Part model, mm, in its own coordinate system. A direction names the side the tool comes from. Round coordinates to 2 decimals unless told otherwise and drop trailing zeros. Order: outer loops, then holes, each group sorted by start corner. A loop starts at its lowest first (then second) coordinate and runs counter-clockwise, first axis right, second up. Notation, with made-up numbers: (57, 66) - (94, 66) arc R22 ccw to (94, 102) - close; hole circle Ø10 at (43.25, -24). An arc over 180 degrees is marked (long way). Return JSON: item names as keys, results as strings. Group by question number.
Item 1: Saw through at B-B on z = 8.25. List the corners of the cut face in (x, y), and give its area (3 significant figures).
Item 2: Saw through at C-C on x = 11.5. List the corners of the cut face in (y, z), and give its area (3 significant figures).
Item 3: Saw through at A-A on y = -59.5. List the corners of the cut face in (x, z), and give its area (3 significant figures).
Item 4: Saw through at D-D on x = -1.5. List the corners of the cut face in (y, z).
Item 5: Probe probe 1 along Y at (x, z) = (24.5, 3.5); probe 2 along Z at (x, y) = (17.5, -43.5); probe 3 along Y at (x, z) = (19, 2.5). List the from-to ranges inside material, lowest first.
Item 6: Drop flat-ended pins along their axis: pin 1 (2 mm diameter, centred on x = 13, z = 4, fed in from +Y); pin 2 (0.5 mm diameter, centred on x = 10.5, y = -0.5, fed in from -Z); pin 3 (0.9 mm diameter, centred on x = 11, y = -92, fed in from +Z); pin 4 (1.3 mm diameter, centred on y = -90.5, z = 8, fed in from -X). Give the stop position or say it passes through.
Item 7: Tool access for faces 4 (the face through (27, -92, 13.048)), 5 (the face through (22, -5, 2)), 6 (the face through (27, -90.5, 8)): list every direction of +Z, -Z, +X, -X, +Y, -Y with a clear straight run to the whole face (end or side of a thin tool).
Item 8: Two-plate mould, pull along X, no slides. Class faces 1 (the face through (17, -53, 0)), 2 (the face through (39.103, -23, 2.5)), 3 (the face through (22.253, -92, 8)): released by +X, released by -X, zero draft, split by the parting line, or undercut.
```python
from build123d import *

# Parameters (mm, degrees)
PAD_DEPTH    = 28
SKETCH002_W  = 44.1
SKETCH002_H  = 3
PAD001_DEPTH = 93.5
PAD002_DEPTH = 5
PAD003_DEPTH = 5
PAD004_DEPTH = 44.1
SKETCH006_W  = 5
SKETCH006_H  = 83.5
POCKET_DEPTH = 5


with BuildPart() as part:
    # Sketch → Pad (new body)
    with BuildSketch(Plane.XY):
        Polygon((-4.997332, 9), (-2.497332, 9), (-2.497332, 8), (-2.997332, 8), (-2.997332, 4), (37.102668, 4), (37.102668, 8), (36.602668, 8), (36.602668, 9), (39.102668, 9), (39.102668, 0), (-4.997332, 0), (-4.997332, 4), align=None)
    extrude(amount=PAD_DEPTH)

    # Sketch002 (on Face11 of Pad) → Pad001 (join)
    with BuildSketch(Plane.XZ):
        with Locations((17.052668, 1.5)):
            Rectangle(SKETCH002_W, SKETCH002_H)
    extrude(amount=PAD001_DEPTH)

    # Sketch003 (on Face18 of Pad001) → Pad002 (join, symmetric)
    with BuildSketch(Plane.YZ.offset(9.102668)):
        Polygon((-93.5, 2.9), (-93.5, 13.04805), (-90.5, 13.04805), (-89.114181, 12.474025), (-90.5, 11.9), (-90.5, 2.9), align=None)
    extrude(amount=PAD002_DEPTH, both=True)

    # Sketch004 (on Face18 of Pad001) → Pad003 (join, symmetric)
    with BuildSketch(Plane.YZ.offset(27.252668)):
        Polygon((-93.5, 2.9), (-93.5, 13.04805), (-90.5, 13.04805), (-89.114181, 12.474025), (-90.5, 11.9), (-90.5, 2.9), align=None)
    extrude(amount=PAD003_DEPTH, both=True)

    # Sketch005 (on Face14 of Pad003) → Pad004 (join)
    with BuildSketch(Plane.YZ.offset(39.102668)):
        Polygon((0.1, 28), (-1.807951, 25), (0.1, 25), align=None)
    extrude(amount=-PAD004_DEPTH)

    # Sketch006 (on Face26 of Pad004) → Pocket (cut)
    with BuildSketch(Plane.XY.offset(3)):
        with Locations((32.328745, -46.75)):
            Rectangle(SKETCH006_W, SKETCH006_H)
        with Locations((2.502668, -46.75)):
            Rectangle(SKETCH006_W, SKETCH006_H)
        with Locations((12.502668, -46.75)):
            Rectangle(SKETCH006_W, SKETCH006_H)
        with Locations((22.502668, -46.75)):
            Rectangle(SKETCH006_W, SKETCH006_H)
    extrude(amount=-POCKET_DEPTH, mode=Mode.SUBTRACT)


solid = part.part
```
Filled in:
{
 "1": {"outline": "(-5, 0) - (39.1, 0) - (39.1, 9) - (36.6, 9) - (36.6, 8) - (37.1, 8) - (37.1, 4) - (-3, 4) - (-3, 8) - (-2.5, 8) - (-2.5, 9) - (-5, 9) - close; (4.1, -93.5) - (14.1, -93.5) - (14.1, -90.5) - (4.1, -90.5) - close; (22.25, -93.5) - (32.25, -93.5) - (32.25, -90.5) - (22.25, -90.5) - close", "area": "257 mm^2"},
 "2": {"outline": "(-93.5, 0) - (-88.5, 0) - (-88.5, 3) - (-90.5, 3) - (-90.5, 11.9) - (-89.11, 12.47) - (-90.5, 13.05) - (-93.5, 13.05) - close; (-5, 0) - (4, 0) - (4, 28) - (0, 28) - (0, 27.84) - (-1.81, 25) - (0, 25) - (0, 3) - (-5, 3) - close", "area": "176 mm^2"},
 "3": {"outline": "(-5, 0) - (0, 0) - (0, 3) - (-5, 3) - close; (5, 0) - (10, 0) - (10, 3) - (5, 3) - close; (15, 0) - (20, 0) - (20, 3) - (15, 3) - close; (25, 0) - (29.83, 0) - (29.83, 3) - (25, 3) - close; (34.83, 0) - (39.1, 0) - (39.1, 3) - (34.83, 3) - close", "area": "72.3 mm^2"},
 "4": {"outline": "(-93.5, 0) - (4, 0) - (4, 28) - (0, 28) - (0, 27.84) - (-1.81, 25) - (0, 25) - (0, 3) - (-93.5, 3) - close"},
 "5": {"probe 1": "y = -93.5 to -90.5, 0 to 4", "probe 2": "z = 0 to 3", "probe 3": "y = -93.5 to 4"},
 "6": {"pin 1": "stops at y = 4", "pin 2": "stops at z = 0", "pin 3": "stops at z = 13.05", "pin 4": "stops at x = 4.1"},
 "7": {"face 4": "+Z, +X, -X, -Y", "face 5": "+Z, -Z", "face 6": "+X, -X"},
 "8": {"face 1": "zero draft", "face 2": "released by +X", "face 3": "undercut"}
}
